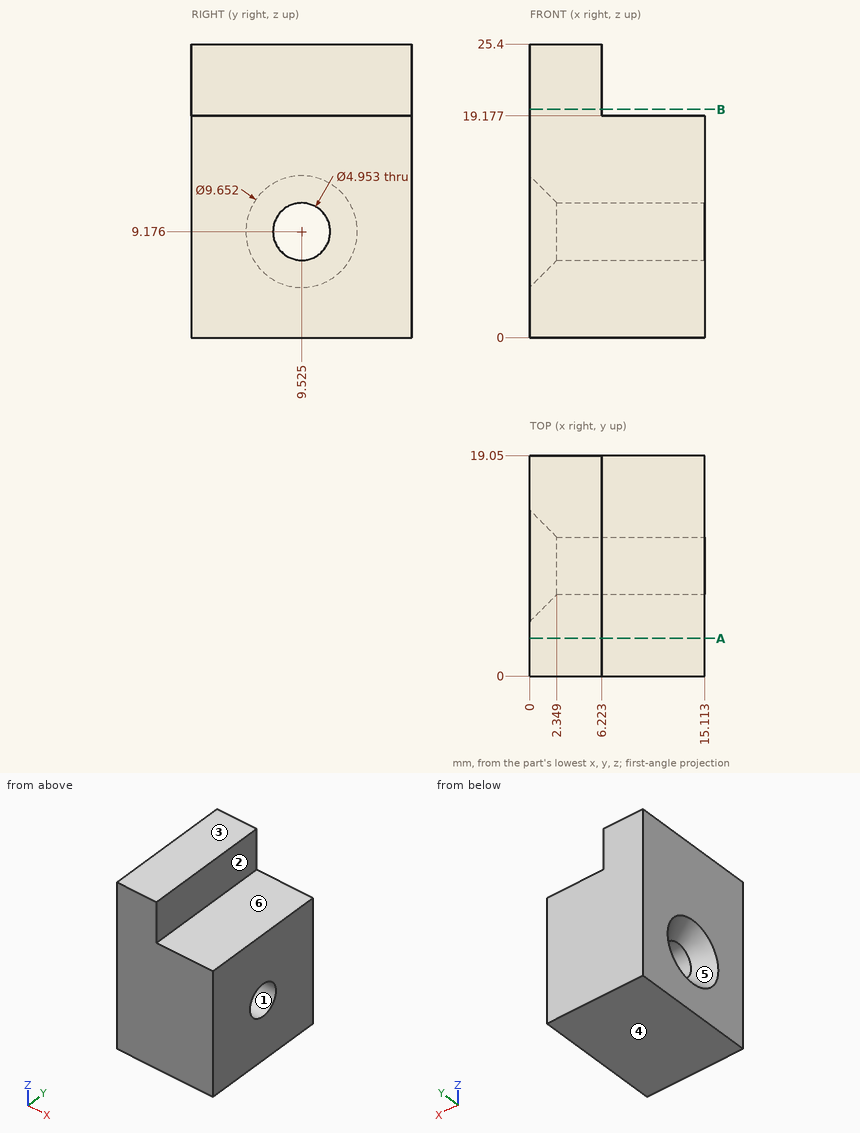
Input: dimensioned drawing with shaded views. Units: mm. Origin: part minimum x, y, z. A direction names the side the tool comes from. Give positions to 0.01 mm unless a question says otherwise; leave off trailing zeros. Loops run counter-clockwise (first coordinate to the right, second up) from the corner with the lowest first, then second, coordinate; pieces in that order, holes last. Notation, with made-up numbers: (28.25, 12) - (83.25, 12) arc R30 ccw to (83.25, 43) - close; hole circle Ø10 at (10, -0.5). An arc over 180 degrees is marked (long way). Answer as CSV lines item,"result". Start each with the question number.
(1) Mould query, pull axis Z, two halves, no side actions, for the marked faces 1, 2, 3 and 4. Classes: +Z half, -Z half, draft (parallel to the pull), parting line (faces both ways), or undercut.
(2) Pin query (flat end, axial travel): P1, Ø1, axis at x = 12.5, y = 11.5, coming from the +Z side; P2, Ø3, axis at y = 7, z = 23, coming from the +X side; P3, Ø4.5, axis at y = 9.52, z = 9.18, coming from the -X side. Return the tip coordinate at first contact, or that it passes through.
(3) Section query B-B (z = 19.75). Output: boundary loops of the cut face in (x, y).
(4) Reachability of the marked faces 5 and 6 from +Z, -Z, +X, -X, +Y, -Y: full face, straight path, thin tool, end or side. Return the list, or none.
(5) Section query A-A (y = 3.25). Output: boundary loops of the cut face in (x, z).
(6) Ray query, line 1 along Z through (x, y) = (14, 6); line 2 along X through (y, z) = (17.75, 21.5); line 3 along Z through (x, y) = (1, 11.25). Return the intervals inside material, ascending. Write a range as [from, to].
Worked answers:
1,face 1,"undercut"
1,face 2,"draft"
1,face 3,"+Z half"
1,face 4,"-Z half"
2,P1,"stops at z = 19.18"
2,P2,"stops at x = 6.22"
2,P3,"passes through"
3,outline,"(0, 0) - (6.22, 0) - (6.22, 19.05) - (0, 19.05) - close"
4,face 5,"-X"
4,face 6,"+Z, +X, +Y, -Y"
5,outline,"(0, 0) - (15.11, 0) - (15.11, 19.18) - (6.22, 19.18) - (6.22, 25.4) - (0, 25.4) - close"
6,line 1,"z = [0, 19.18]"
6,line 2,"x = [0, 6.22]"
6,line 3,"z = [0, 5.76], [12.59, 25.4]"
